Work out the finished part from the listing and answer in its coordinate system (mm). A direction names the side the tool comes from. Round coordinates to 2 decimals unless told otherwise and drop trailing zeros. Order: outer loops, then holes, each group sorted by start corner. A loop starts at its lowest first (then second) coordinate and runs counter-clockwise, first axis right, second up. Notation, with made-up numbers: M -16,36.25 L 19,36.25 A19 ccw 19,45.25 Z; hole C -14.75,44.5 d4. An arc over 180 degrees is marked long. Return JSON: item names as keys, results as strings.
from build123d import *

# Parameters (mm, degrees)
F1_DEPTH = 2.5
F2_R     = 0.85
F3_DEPTH = 12.5


with BuildPart() as f1:
    # F0 (on Top) → F1 (new body)
    with BuildSketch(Plane.XY):
        with BuildLine():
            Line((13.081475452, -13.081475452), (1.0606601718, -1.0606601718))
            ThreePointArc((1.0606601718, -1.0606601718), (0, -0.6213203436), (-1.0606601718, -1.0606601718))
            Line((-1.0606601718, -1.0606601718), (-13.081475452, -13.081475452))
            ThreePointArc((-13.081475452, -13.081475452), (-13.5208152802, -14.1421356237), (-13.081475452, -15.2027957955))
            Line((-13.081475452, -15.2027957955), (-1.0606601718, -27.2236110757))
            ThreePointArc((-1.0606601718, -27.2236110757), (0, -27.6629509039), (1.0606601718, -27.2236110757))
            Line((1.0606601718, -27.2236110757), (13.081475452, -15.2027957955))
            ThreePointArc((13.081475452, -15.2027957955), (13.5208152802, -14.1421356237), (13.081475452, -13.081475452))
        make_face()
        with BuildLine():
            Line((-5.5551142142, -12.6671945862), (-5.5551142142, -7.7095122946))
            Line((-5.5551142142, -7.7095122946), (-4.1542895614, -7.7095122946))
            add(Edge.make_bspline(
                [(-4.1542895614, -7.7095122946), (-3.1679614364, -7.7095122946), (-2.7268807073, -8.0046511835)],
                knots=[0, 0, 0, 1, 1, 1], degree=2))
            add(Edge.make_bspline(
                [(-2.7268807073, -8.0046511835), (-2.2857999781, -8.2997900724), (-2.2857999781, -8.9367258362)],
                knots=[0, 0, 0, 1, 1, 1], degree=2))
            add(Edge.make_bspline(
                [(-2.2857999781, -8.9367258362), (-2.2857999781, -9.3783491001), (-2.5315682073, -9.6648074335)],
                knots=[0, 0, 0, 1, 1, 1], degree=2))
            add(Edge.make_bspline(
                [(-2.5315682073, -9.6648074335), (-2.7773364364, -9.9512657668), (-3.2493416448, -10.0359011835)],
                knots=[0, 0, 0, 1, 1, 1], degree=2))
            Line((-3.2493416448, -10.0359011835), (-3.2493416448, -10.0695383362))
            add(Edge.make_bspline(
                [(-3.2493416448, -10.0695383362), (-2.1197843531, -10.2626806974), (-2.1197843531, -11.2566043085)],
                knots=[0, 0, 0, 1, 1, 1], degree=2))
            add(Edge.make_bspline(
                [(-2.1197843531, -11.2566043085), (-2.1197843531, -11.9206668085), (-2.5690031031, -12.2939306974)],
                knots=[0, 0, 0, 1, 1, 1], degree=2))
            add(Edge.make_bspline(
                [(-2.5690031031, -12.2939306974), (-3.0182218531, -12.6671945862), (-3.8255135198, -12.6671945862)],
                knots=[0, 0, 0, 1, 1, 1], degree=2))
            Line((-3.8255135198, -12.6671945862), (-5.5551142142, -12.6671945862))
        make_face(mode=Mode.SUBTRACT)
        with BuildLine():
            Line((-8.1334756687, -14.8039748892), (-8.1334756687, -13.4802963582))
            Line((-8.1334756687, -13.4802963582), (-0.6236797201, -13.4802963582))
            Line((-0.6236797201, -13.4802963582), (-0.6236797201, -6.9198086858))
            ThreePointArc((-0.6236797201, -6.9198086858), (-0.9032194318, -6.4583786209), (-0.9135835525, -5.9189782686))
            ThreePointArc((-0.9135835525, -5.9189782686), (0.0168397474, -5.0141534426), (0.9868078824, -5.876451129))
            ThreePointArc((0.9868078824, -5.876451129), (0.9900106564, -6.4384308628), (0.6999988109, -6.9198086858))
            Line((0.6999988109, -6.9198086858), (0.6999988109, -13.4802963582))
            Line((0.6999988109, -13.4802963582), (8.1334756687, -13.4802963582))
            ThreePointArc((8.1334756687, -13.4802963582), (8.5949057336, -13.2007566465), (9.134306086, -13.1903925258))
            ThreePointArc((9.134306086, -13.1903925258), (10.0391309119, -14.1208158258), (9.1768332255, -15.0907839607))
            ThreePointArc((9.1768332255, -15.0907839607), (8.6148534917, -15.0939867347), (8.1334756687, -14.8039748892))
            Line((8.1334756687, -14.8039748892), (0.6999988109, -14.8039748892))
            Line((0.6999988109, -14.8039748892), (0.6999988109, -23.1867600232))
            Line((0.6999988109, -23.1867600232), (-0.6236797201, -23.1867600232))
            Line((-0.6236797201, -23.1867600232), (-0.6236797201, -14.8039748892))
            Line((-0.6236797201, -14.8039748892), (-8.1334756687, -14.8039748892))
        make_face(mode=Mode.SUBTRACT)
        Polygon((5.9541938537, -7.5251016937), (5.9541938537, -12.4827839853), (5.3780219787, -12.4827839853), (5.3780219787, -10.1498846798), (2.7662598259, -10.1498846798), (2.7662598259, -12.4827839853), (2.1900879509, -12.4827839853), (2.1900879509, -7.5251016937), (2.7662598259, -7.5251016937), (2.7662598259, -9.6344766937), (5.3780219787, -9.6344766937), (5.3780219787, -7.5251016937), align=None, mode=Mode.SUBTRACT)
    extrude(amount=F1_DEPTH)

    # F2 (on Right) → F3 (cut, symmetric)
    with BuildSketch(Plane.YZ):
        with Locations((-2.4908210296, 1.292226194)):
            Circle(F2_R)
    extrude(amount=F3_DEPTH, both=True, mode=Mode.SUBTRACT)


solid = f1.part
Item 1: Which of the six approach directions +Z, -Z, +X, -X, +Y, -Y give full straight-line access (tool end or side, diameter ignored) to faces 4 (the flat face through (6.987, -21.297, 1.232)), 5 (the cylindrical face through (8.623, -15.096, 1.232))?
Output:
{"face 4": "+Z, -Z, +X, -Y", "face 5": "+Z, -Z"}
Item 2: Find section A-A (y = -5.5). Determine the outline of the cut face in (x, z).
Output:
{"outline": "M -5.5,0 L -0.79,0 L -0.79,2.5 L -5.5,2.5 Z; M 0.87,0 L 5.5,0 L 5.5,2.5 L 0.87,2.5 Z"}
Item 3: The mould has two halves that part along X. Classify faces 1 (the cylindrical face through (-13.52, -14.13, 1.23)), 2 (the flat face through (1, -15, 2.5)), 3 (the flat face through (4, -10.15, 1)): pulls with the +X half, pulls with the -X half, needs draft (parallel to the pull), parting line crosses it, or undercut.
Output:
{"face 1": "pulls with the -X half", "face 2": "needs draft", "face 3": "undercut"}
Item 4: Find section B-B (x = 0.25). Determine the outline of the cut face in (y, z).
Output:
{"outline": "M -27.64,0 L -23.19,0 L -23.19,2.5 L -27.64,2.5 Z; M -5.04,0 L -0.64,0 L -0.64,2.5 L -5.04,2.5 Z; hole C -2.49,1.29 d1.7"}
Item 5: Find section C-C (x = 4). Determine the outline of the cut face in (y, z).
Output:
{"outline": "M -24.28,0 L -14.8,0 L -14.8,2.5 L -24.28,2.5 Z; M -13.48,0 L -10.15,0 L -10.15,2.5 L -13.48,2.5 Z; M -9.63,0 L -4,0 L -4,2.5 L -9.63,2.5 Z"}
Item 6: Find section D-D (z = 0.8). State how many separate pieces and enclosed holes the cut face has, plus the area to 3 significant figures.
Output:
{"separate pieces": "2", "enclosed holes": "3", "area": "321 mm^2"}
Item 7: Each of these flat-tipped pins is pushed along its axis until it touches: pin 1 (0.8 mm diameter, centred on x = -4.5, z = 1.5, fed in from +Y); pin 2 (1.2 mm diameter, centred on y = -10, z = 1.5, fed in from +X); pin 3 (1.2 mm diameter, centred on x = -5, z = 0.5, fed in from -Y). Where does it stop, or does it pass through?
Output:
{"pin 1": "stops at y = -4.1", "pin 2": "stops at x = 10.6", "pin 3": "stops at y = -23.88"}
Item 8: Consider line 1 along Y through (x, z) = (2.5, 1.15); line 2 along Y through (x, z) = (-4.5, 0.6); line 3 along X through (y, z) = (-11, 0.45). Determine where each line is inside the solid, lowest interval first. Write a range as [from, to].
Output:
{"line 1": "y = [-25.78, -14.8], [-13.48, -12.48], [-7.53, -3.33]", "line 2": "y = [-23.78, -14.8], [-13.48, -12.67], [-7.71, -4.5]", "line 3": "x = [-11, -5.56], [-2.14, -0.62], [0.7, 2.19], [2.77, 5.38], [5.95, 11]"}
